Study the drawing (mm; zero at the part's minimum x, y, z) and answer. A direction names the side the tool comes from. Give positions to 0.01 mm unless a question says otherwise; leave off trailing zeros. Write each loop counter-clockwise with the first axis right and the second up, starting at its lowest first coordinate (ties: lowest second). Pieces come first, ordered by that corner, then holes. Notation, with made-up numbers: (18.25, 4.5) - (41.25, 4.5) arc R4 cw to (41.25, 10.5) - close; hole circle Ø11 at (43.5, 1.25). An arc over 180 degrees is marked (long way). One line per item, written item: value. Start each with the question number.
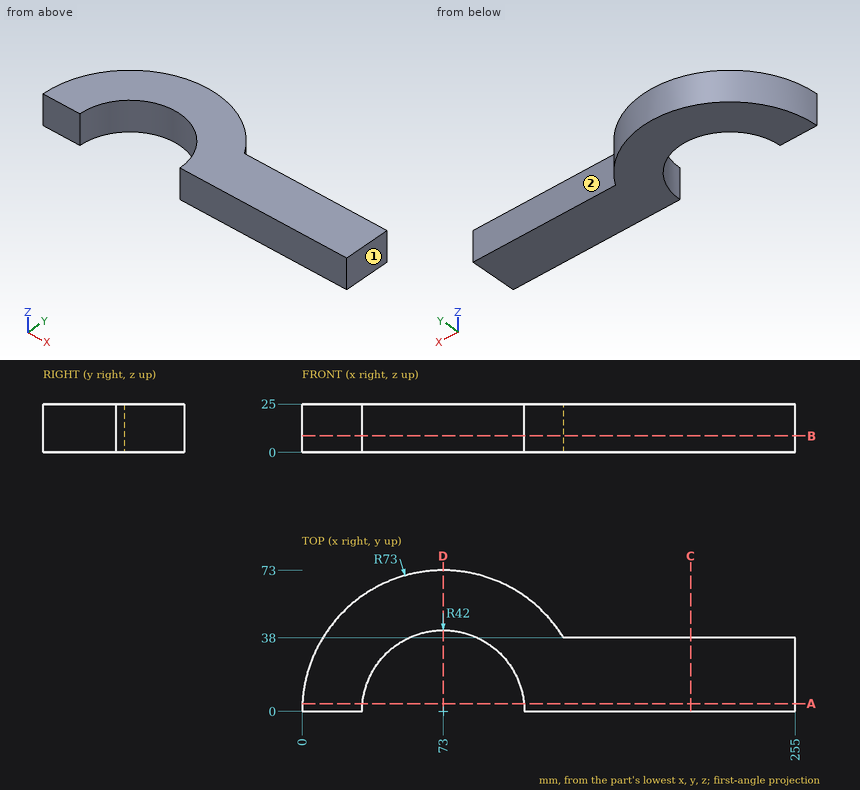
Item 1: Find section B-B on z = 8.5. Determine the outline of the cut face in (x, y), plus the area to 3 significant figures.
Item 2: Find section C-C on x = 201. Determine the outline of the cut face in (y, z).
Item 3: Straight lines are drawn through the part: line 1 along Y through (x, z) = (217.5, 11); line 2 along X through (y, z) = (29.5, 10.5); line 3 along X through (y, z) = (17.5, 20). For each, find the intervals that lie inside material, in ascending order.
Item 4: For the marked faces 1 and 2, determine the directions among +Z, -Z, +X, -X, +Y, -Y from which every point of the face is accessible in a straight line to the end or side of a thin tool.
Item 5: Each of these flat-tipped pins is pushed along its axis until it touches: pin 1 Ø10 at (y, z) = (64, 11) entering from +X; pin 2 Ø4 at (x, z) = (79.5, 16.5) entering from +Y; pin 3 Ø6 at (x, z) = (52.5, 14) entering from -Y. Where does it stop, or does it pass through?
Item 6: Find section D-D on x = 73. Determine the outline of the cut face in (y, z).
Item 7: Find section A-A on y = 4. Determine the outline of the cut face in (x, z).
Values:
1. outline: (0, 0) - (31, 0) arc R42 cw to (115, 0) - (255, 0) - (255, 38) - (135.33, 38) arc R73 ccw to start
1. area: 9,870 mm^2
2. outline: (0, 0) - (38, 0) - (38, 25) - (0, 25) - close
3. line 1: 0 to 38
3. line 2: 6.23 to 43.1, 102.9 to 255
3. line 3: 2.13 to 34.82, 111.18 to 255
4. face 1: +Z, -Z, +X, +Y, -Y
4. face 2: +Z, -Z, +X, +Y
5. pin 1: x = 115.99
5. pin 2: y = 72.86
5. pin 3: y = 34.81
6. outline: (42, 0) - (73, 0) - (73, 25) - (42, 25) - close
7. outline: (0.11, 0) - (31.19, 0) - (31.19, 25) - (0.11, 25) - close; (114.81, 0) - (255, 0) - (255, 25) - (114.81, 25) - close
